```python
from build123d import *

# Parameters (mm, degrees)
SKETCH1_W           = 4.7625
SKETCH1_H           = 26.974800888
SKETCH1_H_2         = 26.974800889
BOSS_EXTRUDE1_DEPTH = 4.7625


with BuildPart() as part:
    # Sketch1 → Boss-Extrude1 (new body)
    with BuildSketch(Plane.XY):
        Polygon((65.88125, 142.515737536), (127, 142.515737536), (127, 15.515737536), (0, 15.515737536), (0, 142.515737536), (61.11875, 142.515737536), align=None)
        with Locations((8.73125, 103.628337092)):
            Rectangle(SKETCH1_W, SKETCH1_H, mode=Mode.SUBTRACT)
        with Locations((118.26875, 103.628337092)):
            Rectangle(SKETCH1_W, SKETCH1_H, mode=Mode.SUBTRACT)
        with Locations((118.26875, 54.403137981)):
            Rectangle(SKETCH1_W, SKETCH1_H_2, mode=Mode.SUBTRACT)
        with Locations((8.73125, 54.403137981)):
            Rectangle(SKETCH1_W, SKETCH1_H_2, mode=Mode.SUBTRACT)
    extrude(amount=BOSS_EXTRUDE1_DEPTH)


solid = part.part
```
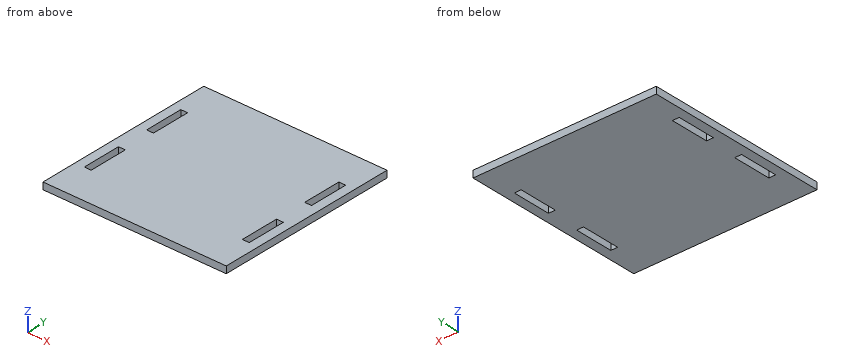
Can you work these out from the model? Positions are in its coordinate system, mm. Round coordinates to 2 decimals unless told otherwise and drop trailing zeros. Loops run counter-clockwise (first coordinate to the right, second up) from the corner with the lowest first, then second, coordinate; pieces in that order, holes last. Notation, with made-up numbers: (10, -35.5) -> (49, -35.5) arc R14 cw to (49, -17.5) -> close; hole circle Ø6 at (-37, 27.25). An arc over 180 degrees is marked (long way). One line per item, written item: value. Start each with the question number.
1. If I drill on probe 1 along Y at (x, z) = (120, 1.4); probe 2 along X at (y, z) = (103, 0.35), over which ranges is the centre line in solid material (lowest first)?
2. If we section it at B-B, the plane z = 1.5: Write out the boundary of the cut face in (x, y), then the cut area to 3 significant figures.
3. If we section it at A-A, the plane y = 48: Write out the boundary of the cut face in (x, z), then the cut area to 3 significant figures.
Calculated:
1. probe 1: y = 15.52 to 40.92, 67.89 to 90.14, 117.12 to 142.52
1. probe 2: x = 0 to 6.35, 11.11 to 115.89, 120.65 to 127
2. outline: (0, 15.52) -> (127, 15.52) -> (127, 142.52) -> (0, 142.52) -> close; hole (6.35, 40.92) -> (11.11, 40.92) -> (11.11, 67.89) -> (6.35, 67.89) -> close; hole (6.35, 90.14) -> (11.11, 90.14) -> (11.11, 117.12) -> (6.35, 117.12) -> close; hole (115.89, 40.92) -> (120.65, 40.92) -> (120.65, 67.89) -> (115.89, 67.89) -> close; hole (115.89, 90.14) -> (120.65, 90.14) -> (120.65, 117.12) -> (115.89, 117.12) -> close
2. area: 15,600 mm²
3. outline: (0, 0) -> (6.35, 0) -> (6.35, 4.76) -> (0, 4.76) -> close; (11.11, 0) -> (115.89, 0) -> (115.89, 4.76) -> (11.11, 4.76) -> close; (120.65, 0) -> (127, 0) -> (127, 4.76) -> (120.65, 4.76) -> close
3. area: 559 mm²
